The model under review builds one solid part; all positions refer to its coordinate system, in mm. Face numbers are marked on the shaded views. A direction names the side the tool comes from. Round coordinates to 2 decimals unless told otherwise and drop trailing zeros. Write each loop counter-clockwise with the first axis right and the second up, starting at its lowest first coordinate (ties: lowest second). Pieces come first, ordered by that corner, then holes. Notation, with made-up numbers: (47.25, 64) - (62.25, 64) arc R29 cw to (62.25, 91) - close; hole circle Ø3 at (49, 75.25). An arc over 180 degrees is marked (long way). Use one line per item in the form item = value.
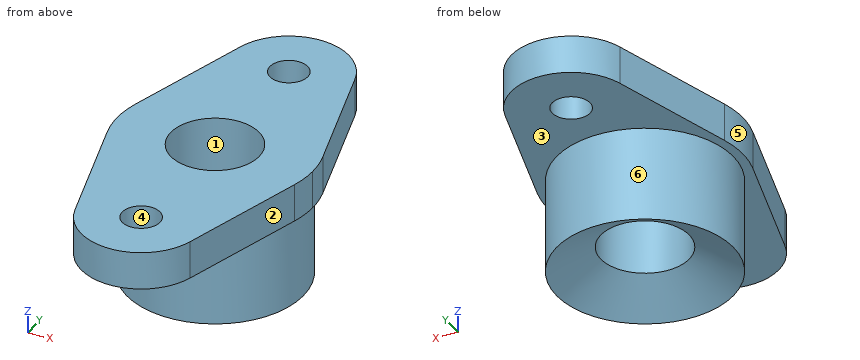
from build123d import *

# Parameters (mm, degrees)
F0_R     = 6
F0_R_2   = 14
F1_DEPTH = 12
F2_R     = 28
F2_R_2   = 14
F3_DEPTH = 30


with BuildPart() as f1:
    # F0 (on Top) → F1 (new body)
    with BuildSketch(Plane.XY):
        with BuildLine():
            ThreePointArc((11.4242022345, 28.8181818182), (17.0008800133, 35.5164819342), (19, 44))
            ThreePointArc((19, 44), (18.8190726431, 46.6158182), (18.279736331, 49.1818181818))
            ThreePointArc((18.279736331, 49.1818181818), (0, 63), (-18.279736331, 49.1818181818))
            ThreePointArc((-18.279736331, 49.1818181818), (-18.0069545749, 37.9378562425), (-11.4242022345, 28.8181818182))
            ThreePointArc((-11.4242022345, 28.8181818182), (0, 31), (11.4242022345, 28.8181818182))
        make_face()
        with Locations((0, 44)):
            Circle(F0_R, mode=Mode.SUBTRACT)
        with BuildLine():
            ThreePointArc((-11.4242022345, 28.8181818182), (-18.0069545749, 37.9378562425), (-18.279736331, 49.1818181818))
            Line((-18.279736331, 49.1818181818), (-29.8248329611, 8.4545454545))
            ThreePointArc((-29.8248329611, 8.4545454545), (-23.000872758, 20.7836438665), (-11.4242022345, 28.8181818182))
        make_face()
        with BuildLine():
            ThreePointArc((18.279736331, 49.1818181818), (18.8190726431, 46.6158182), (19, 44))
            ThreePointArc((19, 44), (17.0008800133, 35.5164819342), (11.4242022345, 28.8181818182))
            ThreePointArc((11.4242022345, 28.8181818182), (23.000872758, 20.7836438665), (29.8248329611, 8.4545454545))
            Line((29.8248329611, 8.4545454545), (18.279736331, 49.1818181818))
        make_face()
        with BuildLine():
            ThreePointArc((-11.4242022345, 28.8181818182), (0, 25), (11.4242022345, 28.8181818182))
            ThreePointArc((11.4242022345, 28.8181818182), (0, 31), (-11.4242022345, 28.8181818182))
        make_face()
        with BuildLine():
            ThreePointArc((29.8248329611, 8.4545454545), (23.000872758, 20.7836438665), (11.4242022345, 28.8181818182))
            ThreePointArc((11.4242022345, 28.8181818182), (0, 25), (-11.4242022345, 28.8181818182))
            ThreePointArc((-11.4242022345, 28.8181818182), (-23.000872758, 20.7836438665), (-29.8248329611, 8.4545454545))
            ThreePointArc((-29.8248329611, 8.4545454545), (-31, 0), (-29.8248329611, -8.4545454545))
            ThreePointArc((-29.8248329611, -8.4545454545), (-23.000872758, -20.7836438665), (-11.4242022345, -28.8181818182))
            ThreePointArc((-11.4242022345, -28.8181818182), (0, -25), (11.4242022345, -28.8181818182))
            ThreePointArc((11.4242022345, -28.8181818182), (23.000872758, -20.7836438665), (29.8248329611, -8.4545454545))
            ThreePointArc((29.8248329611, -8.4545454545), (30.7048027334, -4.2679139053), (31, 0))
            ThreePointArc((31, 0), (30.7048027334, 4.2679139053), (29.8248329611, 8.4545454545))
        make_face()
        Circle(F0_R_2, mode=Mode.SUBTRACT)
        with BuildLine():
            ThreePointArc((11.4242022345, -28.8181818182), (0, -25), (-11.4242022345, -28.8181818182))
            ThreePointArc((-11.4242022345, -28.8181818182), (0, -31), (11.4242022345, -28.8181818182))
        make_face()
        with BuildLine():
            ThreePointArc((-11.4242022345, -28.8181818182), (-23.000872758, -20.7836438665), (-29.8248329611, -8.4545454545))
            Line((-29.8248329611, -8.4545454545), (-18.279736331, -49.1818181818))
            ThreePointArc((-18.279736331, -49.1818181818), (-18.0069545749, -37.9378562425), (-11.4242022345, -28.8181818182))
        make_face()
        with BuildLine():
            Line((18.279736331, -49.1818181818), (29.8248329611, -8.4545454545))
            ThreePointArc((29.8248329611, -8.4545454545), (23.000872758, -20.7836438665), (11.4242022345, -28.8181818182))
            ThreePointArc((11.4242022345, -28.8181818182), (17.0008800133, -35.5164819342), (19, -44))
            ThreePointArc((19, -44), (18.8190726431, -46.6158182), (18.279736331, -49.1818181818))
        make_face()
        with BuildLine():
            ThreePointArc((11.4242022345, -28.8181818182), (0, -31), (-11.4242022345, -28.8181818182))
            ThreePointArc((-11.4242022345, -28.8181818182), (-18.0069545749, -37.9378562425), (-18.279736331, -49.1818181818))
            ThreePointArc((-18.279736331, -49.1818181818), (0, -63), (18.279736331, -49.1818181818))
            ThreePointArc((18.279736331, -49.1818181818), (18.8190726431, -46.6158182), (19, -44))
            ThreePointArc((19, -44), (17.0008800133, -35.5164819342), (11.4242022345, -28.8181818182))
        make_face()
        with Locations((0, -44)):
            Circle(F0_R, mode=Mode.SUBTRACT)
    extrude(amount=F1_DEPTH)

    # F2 (on face) → F3 (join)
    with BuildSketch(Plane(origin=(0, 0, 0), x_dir=(1, 0, 0), z_dir=(0, 0, -1))):
        Circle(F2_R)
        Circle(F2_R_2, mode=Mode.SUBTRACT)
    extrude(amount=F3_DEPTH)

    # F4 (on Front) → F5 (revolve, cut)
    with BuildSketch(Plane.XZ):
        Polygon((28, -30), (14, -21.9170962313), (14, -30), align=None)
    revolve(axis=Axis((0, 0, -30), (0, 0, -1)), mode=Mode.SUBTRACT)


solid = f1.part
(1) Machinability: for the marked faces 5 and 6, which of the approach directions +Z, -Z, +X, -X, +Y, -Y give a long, thin tool a straight path to every point of the face, cutting with its end or side? Answer none if there is none.
Geometry results:
face_5 = +Z, -Z, -X
face_6 = -Z
(2) Insertion check: P1, Ø6, axis at x = 17, y = -26.5, coming from the -Z side; P2, Ø2, axis at y = 33.5, z = 4.5, coming from the -X side; P3, Ø6, axis at x = -16.5, y = 18.5, coming from the -Z side; P4, Ø17, axis at x = 0, y = 0, coming from the -Z side. Each pin has a flat end and moves straight along its axis. Give the tip position at first contact, or say it passes through.
Geometry results:
P1 = 0
P2 = -23.01
P3 = -29.88
P4 = through
(3) Add section D-D on y = 55. Write out the cut boundary in (x, z), then the cut area to 3 significant figures.
Geometry results:
outline = (-15.49, 0) - (15.49, 0) - (15.49, 12) - (-15.49, 12) - close
area = 372 mm2
(4) Add section A-A on x = 0. Write out the cut boundary in (y, z), then the cut area to 3 significant figures.
Geometry results:
outline = (-63, 0) - (-50, 0) - (-50, 12) - (-63, 12) - close; (-38, 0) - (-28, 0) - (-28, -30) - (-14, -21.92) - (-14, 12) - (-38, 12) - close; (14, -21.92) - (28, -30) - (28, 0) - (38, 0) - (38, 12) - (14, 12) - close; (50, 0) - (63, 0) - (63, 12) - (50, 12) - close
area = 1,610 mm2
(5) Add section C-C on z = -3. Write out the cut boundary in (x, y).
Geometry results:
outline = circle Ø56 at (0, 0); hole circle Ø28 at (0, 0)
(6) To check wall thickness, follow L1, parallel to Y at x = 0, z = 8.5; L2, parallel to Y at x = 0, z = -12; L3, parallel to Z at x = -27, y = -11. State the ranges of each line that lie inside material, in increasing order.
Geometry results:
L1 = -63 to -50, -38 to -14, 14 to 38, 50 to 63
L2 = -28 to -14, 14 to 28
L3 = 0 to 12
(7) Add section B-B on y = -44. Write out the cut boundary in (x, z), then the cut area to 3 significant figures.
Geometry results:
outline = (-19.75, 0) - (-6, 0) - (-6, 12) - (-19.75, 12) - close; (6, 0) - (19.75, 0) - (19.75, 12) - (6, 12) - close
area = 330 mm2
(8) The part is to be moulded in two halves that separate along Y. For the marked faces 1, 2, 3 and 4, say which applies: +Y half, -Y half, draft (parallel to the pull), parting line (faces both ways), or undercut.
Geometry results:
face_1 = undercut
face_2 = -Y half
face_3 = draft
face_4 = undercut
